Could you check a few things on this model? Use its own coordinates, in mm. A direction names the side the tool comes from. Round coordinates to 2 decimals unless told otherwise and drop trailing zeros. Loops run counter-clockwise (first coordinate to the right, second up) from the corner with the lowest first, then second, coordinate; pieces in that order, holes last.
from build123d import *

# Parameters (mm, degrees)
SKETCH_1_R          = 24
SKETCH_1_R_2        = 19
EXTRUDE_1_DEPTH     = 10
SKETCH_2_R          = 25
SKETCH_2_R_2        = 19
EXTRUDE_2_DEPTH     = 20
CUT_EXTRUDE_1_DEPTH = 31
SKETCH_4_R          = 21
CUT_EXTRUDE_2_DEPTH = 7
CHAMFER_1_SIZE      = 0.6


with BuildPart() as part:
    # 草图1 → 凸台-拉伸1 (new body)
    with BuildSketch(Plane(origin=(0, 0, 0), x_dir=(1, 0, 0), z_dir=(0, 1, 0))):
        Circle(SKETCH_1_R)
        Circle(SKETCH_1_R_2, mode=Mode.SUBTRACT)
    extrude(amount=EXTRUDE_1_DEPTH)

    # 草图2 → 凸台-拉伸2 (add)
    with BuildSketch(Plane(origin=(0, 10, 0), x_dir=(1, 0, 0), z_dir=(0, 1, 0))):
        Circle(SKETCH_2_R)
        Circle(SKETCH_2_R_2, mode=Mode.SUBTRACT)
    extrude(amount=EXTRUDE_2_DEPTH)

    # 草图3 → 切除-拉伸1 (cut, symmetric)
    with BuildSketch(Plane(origin=(0, 0, 0), x_dir=(0, 0, -1), z_dir=(1, 0, 0))):
        Polygon((-25, 17), (25, 25.816349035), (25, 47.879470908), (-25, 47.879470908), align=None)
    extrude(amount=CUT_EXTRUDE_1_DEPTH, both=True, mode=Mode.SUBTRACT)

    # 草图4 → 切除-拉伸2 (cut)
    with BuildSketch(Plane(origin=(0, 20.762639068, 3.661013458), x_dir=(1, 0, 0), z_dir=(0, 0.984807753, 0.173648178))):
        with Locations((0, 3.717490492)):
            Circle(SKETCH_4_R)
    extrude(amount=-CUT_EXTRUDE_2_DEPTH, mode=Mode.SUBTRACT)

    # 倒角1
    chamfer_1_edges = [part.edges().sort_by_distance(p)[0] for p in [
        (-21, 21.408174518, 0),
    ]]
    chamfer(chamfer_1_edges, length=CHAMFER_1_SIZE)


solid = part.part
Item 1: For faces 1 (the cylindrical face through (-3.255, 16.04, -24.787)), 2 (the flat face through (-9.4, 10, -22.3)), which set-ups out of +Z, -Z, +X, -X, +Y, -Y let a thin tool reach every point of the face, with its end or its side?
Results list:
face 1: +Y, -Y
face 2: -Y
Item 2: We'd pull the mould along X, two halves only. Please class faces 3 (the flat face through (20.487, 20.081, 7.524)), 4 (the cylindrical face through (9.69, 14.475, 17.695)), 5 (the cylindrical face through (-23.977, 4.93, -1.055)), 6 (the flat face through (-0.098, 17.773, -19.695)): released by +X, released by -X, zero draft, split by the parting line, or undercut.
Results list:
face 3: zero draft
face 4: undercut
face 5: split by the parting line
face 6: undercut
Item 3: Will these pins go through, and if not, where does the flat tip stop? pin 1 (12 mm diameter, centred on x = -19, y = 12.5, fed in from -Z); pin 2 (1 mm diameter, centred on y = 15, z = 14, fed in from +X); pin 3 (5 mm diameter, centred on y = 17, z = 10, fed in from -X).
Results list:
pin 1: stops at z = -21.35
pin 2: stops at x = 21.04
pin 3: stops at x = -23.85
Item 4: If we section it at A-A, the plane y = 2.5: Please give me the cut outline in (x, z).
Results list:
outline: circle Ø48 at (0, 0); hole circle Ø38 at (0, 0)
Item 5: If I drill on line 1 along X through (y, z) = (13, 0); line 2 along Z through (x, y) = (0, 8), over which ranges is the centre line in solid material (lowest first)?
Results list:
line 1: x = -25 to -19, 19 to 25
line 2: z = -24 to -19, 19 to 24
